Work out the finished part from the listing and answer in its coordinate system (mm). Face numbers are marked on the shaded views. A direction names the side the tool comes from. Coordinates: 2 decimals unless noted, no trailing zeros. Order: outer loops, then holes, each group sorted by start corner. A loop starts at its lowest first (then second) coordinate and runs counter-clockwise, first axis right, second up. Notation, with made-up numbers: M 74,50.5 L 105,50.5 A28 ccw 105,80.5 Z; hole C 44.25,-27 d3. An arc over 180 degrees is marked long. Use a Markdown table: item, result.
from build123d import *

# Parameters (mm, degrees)
SKETCH1_R           = 5
BOSS_EXTRUDE1_DEPTH = 5
SKETCH2_R           = 2.5
CUT_EXTRUDE1_DEPTH  = 2.5
SKETCH3_R           = 1.25
CUT_EXTRUDE2_DEPTH  = 9.660254038
CHAMFER1_SIZE       = 2.5


with BuildPart() as part:
    # Sketch1 → Boss-Extrude1 (new body)
    with BuildSketch(Plane.XY):
        Circle(SKETCH1_R)
    extrude(amount=BOSS_EXTRUDE1_DEPTH)

    # Sketch2 → Cut-Extrude1 (cut)
    with BuildSketch(Plane.XY.offset(5)):
        Circle(SKETCH2_R)
    extrude(amount=-CUT_EXTRUDE1_DEPTH, mode=Mode.SUBTRACT)

    # Sketch3 → Cut-Extrude2 (cut, through all)
    with BuildSketch(Plane(origin=(0, 0, 0), x_dir=(-1, 0, 0), z_dir=(0, 0, -1))):
        Circle(SKETCH3_R)
    extrude(amount=-CUT_EXTRUDE2_DEPTH, mode=Mode.SUBTRACT)

    # Chamfer1
    chamfer1_edges = [part.edges().sort_by_distance(p)[0] for p in [
        (-5, 0, 0),
    ]]
    chamfer(chamfer1_edges, length=CHAMFER1_SIZE)


solid = part.part
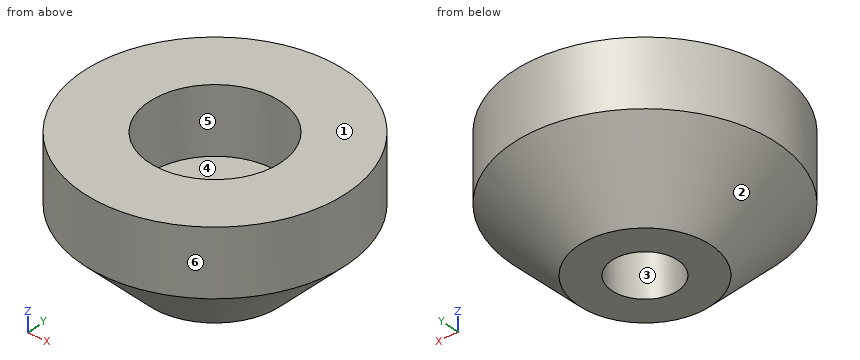
(1) A cutting plane is placed at C-C (z = 1.3). Determine the outline of the cut face in (x, y).
Conclusion:
| item | result |
|---|---|
| outline | C 0,0 d7.6; hole C 0,0 d2.5 |
(2) Given P1, Ø2, axis at x = -3, z = 1, coming from the -Y side; P2, Ø1.5, axis at x = 0.5, y = 0.5, coming from the +Z side, each flat-ended and moving along its own axis, determine where each tip first touches the part or whether it passes through.
Conclusion:
| item | result |
|---|---|
| P1 | y = -3.58 |
| P2 | z = 2.5 |
(3) Straight lines are drawn through the part: L1, parallel to Y at x = 0, z = 4.45; L2, parallel to Z at x = -1, y = -1; L3, parallel to Y at x = -0.5, z = 0.7. For each, find the intervals that lie inside material, in ascending order.
Conclusion:
| item | result |
|---|---|
| L1 | -5 to -2.5, 2.5 to 5 |
| L2 | 0 to 2.5 |
| L3 | -3.16 to -1.15, 1.15 to 3.16 |
(4) A cutting plane is placed at A-A (x = 0). Determine the outline of the cut face in (y, z), then the cut area to 3 significant figures.
Conclusion:
| item | result |
|---|---|
| outline | M -5,2.5 L -2.5,0 L -1.25,0 L -1.25,2.5 L -2.5,2.5 L -2.5,5 L -5,5 Z; M 1.25,0 L 2.5,0 L 5,2.5 L 5,5 L 2.5,5 L 2.5,2.5 L 1.25,2.5 Z |
| area | 25.0 mm2 |
(5) Determine the mould class of the marked faces 1, 2, 3 and 4 for opening direction X: pulls with the +X half, pulls with the -X half, needs draft (parallel to the pull), parting line crosses it, or undercut.
Conclusion:
| item | result |
|---|---|
| face 1 | needs draft |
| face 2 | parting line crosses it |
| face 3 | undercut |
| face 4 | undercut |
(6) Which of the six approach directions +Z, -Z, +X, -X, +Y, -Y give full straight-line access (tool end or side, diameter ignored) to the marked faces 5 and 6?
Conclusion:
| item | result |
|---|---|
| face 5 | +Z |
| face 6 | +Z, -Z |
